from build123d import *

# Parameters (mm, degrees)
BOSS_EXTRUDE2_DEPTH = 90
BOSS_EXTRUDE4_DEPTH = 10
BOSS_EXTRUDE5_DEPTH = 10
FILLET1_R           = 10


with BuildPart() as part:
    # Sketch1 → Boss-Extrude2 (new body)
    with BuildSketch(Plane(origin=(0, 0, 0), x_dir=(0, 0, -1), z_dir=(1, 0, 0))):
        with BuildLine():
            Line((-48.118811881, 0), (41.881188119, 0))
            Line((41.881188119, 0), (41.881188119, 83.466961913))
            Line((41.881188119, 83.466961913), (27.086166787, 83.466961913))
            ThreePointArc((27.086166787, 83.466961913), (24.257739663, 82.295389038), (23.086166787, 79.466961913))
            Line((23.086166787, 79.466961913), (23.086166787, 32.998967786))
            ThreePointArc((23.086166787, 32.998967786), (13.24711535, 23.473123138), (0, 20))
            Line((0, 20), (-48.118811881, 20))
            Line((-48.118811881, 20), (-48.118811881, 0))
        make_face()
    extrude(amount=-BOSS_EXTRUDE2_DEPTH)

    # Sketch2 → Boss-Extrude4 (add, symmetric)
    with BuildSketch(Plane(origin=(0, 0, 0), x_dir=(0, 0, -1), z_dir=(1, 0, 0))):
        with BuildLine():
            Line((-32.487137017, 0), (-51.053894903, -25.643291777))
            Line((-51.053894903, -25.643291777), (-39.969263329, -25.643291777))
            Line((-39.969263329, -25.643291777), (-23.065200179, 0))
            Line((-23.065200179, 0), (10.956889222, 0))
            Line((10.956889222, 0), (22.448464713, -25.643291777))
            Line((22.448464713, -25.643291777), (35.102344658, -25.643291777))
            Line((35.102344658, -25.643291777), (22.448464713, 0))
            Line((22.448464713, 0), (17.947936645, 9.120392711))
            ThreePointArc((17.947936645, 9.120392711), (-3.967837589, 4.007448958), (-25.883611823, 9.120392711))
            Line((-25.883611823, 9.120392711), (-32.487137017, 0))
        make_face()
    extrude(amount=BOSS_EXTRUDE4_DEPTH, both=True)

    # Sketch5 → Boss-Extrude5 (add, symmetric)
    with BuildSketch(Plane.ZY.offset(90)):
        Polygon((-15.060305743, 7.399353966), (28.775027298, 7.399353966), (50.037353524, -23.467201706), (39.406190411, -23.467201706), (21.793994687, 0), (-13.237941151, 0), (-23.164531139, -23.467201706), (-36.584121335, -23.467201706), (-21.202482156, 7.399353966), align=None)
    extrude(amount=BOSS_EXTRUDE5_DEPTH, both=True)

    # Fillet1
    fillet1_edges = [part.edges().sort_by_distance(p)[0] for p in [
        (-95, 7.399353966, 28.775027298),
        (-95, 7.399353966, -21.202482156),
    ]]
    fillet(fillet1_edges, radius=FILLET1_R)


solid = part.part
Build history of the part. All positions in model axes, mm. A direction names the side the tool comes from. Round coordinates to 2 decimals unless told otherwise and drop trailing zeros. Write each loop counter-clockwise with the first axis right and the second up, starting at its lowest first coordinate (ties: lowest second). Pieces come first, ordered by that corner, then holes. Notation, with made-up numbers: (-33, 26.5) - (12, 26.5) arc R20 cw to (12, 57.5) - close; hole circle Ø7 at (77.5, 14.5). An arc over 180 degrees is marked (long way). One line per question, with ' | ' between items.
1. Band-saw the part on D-D, the plane z = -3. Write the cut outline in (x, y), and give its area (3 significant figures).
Results are:
outline: (-100, 0) - (10, 0) - (10, 4.5) - (0, 4.5) - (0, 20.17) - (-90, 20.17) - (-90, 7.4) - (-100, 7.4) - close | area: 1,930 mm^2
2. Drill centre lines: line 1 along Y through (x, z) = (-59.5, -33); line 2 along Y through (x, z) = (-35, 16.5); line 3 along Z through (x, y) = (-56.5, 65). Where is each one in solid material? Low to high. Write a range as from..to.
Results are:
line 1: 0..83.47 | line 2: 0..20 | line 3: -41.88..-23.09
3. Band-saw the part on A-A, the plane x = -64. Write the cut outline in (y, z), and give its area (3 significant figures).
Results are:
outline: (0, -41.88) - (83.47, -41.88) - (83.47, -27.09) arc R4 ccw to (79.47, -23.09) - (33, -23.09) arc R27 cw to (20, 0) - (20, 48.12) - (0, 48.12) - close | area: 3,080 mm^2
4. Tool access for faces 1 (the face through (0, 24, -16)), 2 (the face through (-10, -13, -23)), 3 (the face through (-90.14, -11.57, -18.13)): list every direction of +Z, -Z, +X, -X, +Y, -Y with a clear straight run to the whole face (end or side of a thin tool).
Results are:
face 1: +X, +Y | face 2: +Z, -Z, -Y | face 3: -X, -Y
5. Band-saw the part on B-B, the plane z = 36. Write the cut outline in (x, y).
Results are:
outline: (-100, -18.93) - (-80, -18.93) - (-80, -3.09) - (-100, -3.09) - close; (-90, 0) - (0, 0) - (0, 20) - (-90, 20) - close; (-10, -19.62) - (10, -19.62) - (10, -4.85) - (-10, -4.85) - close
6. Band-saw the part on C-C, the plane y = -12.5. Write the cut outline in (x, z), and give its area (3 significant figures).
Results are:
outline: (-100, -31.12) - (-80, -31.12) - (-80, -18.53) - (-100, -18.53) - close; (-100, 31.18) - (-80, 31.18) - (-80, 42.48) - (-100, 42.48) - close; (-10, -28.62) - (10, -28.62) - (10, -16.56) - (-10, -16.56) - close; (-10, 31.31) - (10, 31.31) - (10, 41.54) - (-10, 41.54) - close | area: 924 mm^2
7. Drop flat-ended pins along their axis: pin 1 Ø5 at (y, z) = (10, 12.5) entering from +X; pin 2 Ø8 at (x, z) = (-12, 11.5) entering from -Y; pin 3 Ø1 at (x, z) = (-81, 33) entering from +Y. Give the stop position or say it passes through.
Results are:
pin 1: x = 0 | pin 2: y = 0 | pin 3: y = 20
8. Mould opens along Z. For faces 4 (the face through (0.14, -13.001, 31.636)), 5 (the face through (-44, 10, 48.119)), 6 (the face through (0.14, -12.64, -16.62)), 7 (the face through (-95.07, 5.943, -20.21)) say: released by +Z, released by -Z, zero draft, split by the parting line, or undercut.
Results are:
face 4: undercut | face 5: released by +Z | face 6: undercut | face 7: released by -Z
